For this review, take the finished solid that the model builds, in its own axes (mm). Face numbers are marked on the shaded views. Give positions to 0.01 mm unless a question says otherwise; leave off trailing zeros. Loops run counter-clockwise (first coordinate to the right, second up) from the corner with the lowest first, then second, coordinate; pieces in that order, holes last. Notation, with made-up numbers: (61, -10.75) - (101, -10.75) arc R29 ccw to (101, 11.25) - close; hole circle Ø1 at (-9, 22). An arc over 180 degrees is marked (long way). Put each result on its own line as item: value. Start each with the question number.
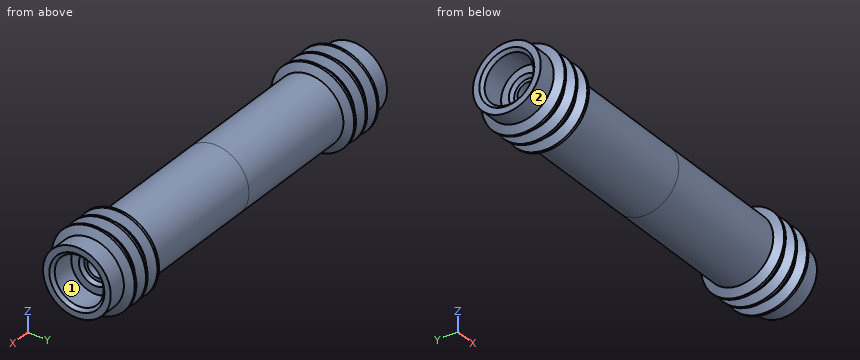
from build123d import *

# Parameters (mm, degrees)
CHAMFER1_SIZE = 0.508


with BuildPart() as part:
    # Sketch2 → Revolve1 (revolve)
    with BuildSketch(Plane.XY, mode=Mode.PRIVATE) as revolve1_sk:
        Polygon((-28.75, 5.55625), (-31.75, 5.55625), (-31.75, 4), (-27.45, 4), (-27.45, 2.73), (-26.942, 2.222), (-26.942, 1.7145), (-21.925, 1.7145), (-21.925, 0), (0, 0), (0, 3.175), (0, 5.55625), (-21.705060633, 5.55625), (-22.438295474, 6.82625), (-22.819295474, 6.82625), (-23.552530316, 5.55625), (-24.314530316, 5.55625), (-25.047765158, 6.82625), (-25.428765158, 6.82625), (-26.162, 5.55625), (-26.924, 5.55625), (-27.657234842, 6.82625), (-28.016765158, 6.82625), align=None)
    revolve(revolve1_sk.sketch.rotate(Axis((-31.75, 0, 0), (1, 0, 0)), 180), axis=Axis((-31.75, 0, 0), (1, 0, 0)))

    # Chamfer1
    chamfer1_edges = [part.edges().sort_by_distance(p)[0] for p in [
        (-31.75, 4, 0),
    ]]
    chamfer(chamfer1_edges, length=CHAMFER1_SIZE)

    # Mirror1: part across plane


with BuildPart() as part_1:
    add(part.part)
    add(part.part.mirror(Plane(origin=(0, 0, 0), x_dir=(0, 0, 1), z_dir=(1, 0, 0))))


solid = part_1.part
1) Wall thickness on probe 1 along X at (y, z) = (1.25, 6); probe 2 along Y at (x, z) = (-28, -0.25); probe 3 along X at (y, z) = (3, -6): over which ranges is each line inside the solid? List them lowest first.
2) Mouldability with a two-part tool opening along Z and no side actions: class the marked faces 1 and 2 as released by +Z, released by -Z, zero draft, split by the parting line, or undercut.
3) Take a section at A-A on x = -9.5. State the section outline as (y, z) points.
4) Insertion check: P1, Ø6, axis at x = 13, z = -2, coming from the +Y side; P2, Ø8, axis at x = -18, z = -4.5, coming from the +Y side; P3, Ø5, axis at y = 1, z = 0, coming from the -X side. Each pin has a flat end and moves straight along its axis. Give the tip position at first contact, or say it passes through.
Answers follow:
1. probe 1: -28.42 to -27.25, -25.83 to -24.65, -23.22 to -22.04, 22.04 to 23.22, 24.65 to 25.83, 27.25 to 28.42
1. probe 2: -6.82 to -3.99, 3.99 to 6.82
1. probe 3: -28.08 to -27.59, -25.5 to -24.98, -22.89 to -22.37, 22.37 to 22.89, 24.98 to 25.5, 27.59 to 28.08
2. face 1: undercut
2. face 2: split by the parting line
3. outline: circle Ø11.11 at (0, 0)
4. P1: y = 5.56
4. P2: y = 5.53
4. P3: x = -27.45
